Could you check a few things on this model? Use its own coordinates, in mm. A direction names the side the tool comes from. Coordinates: 2 decimals unless noted, no trailing zeros. Write each loop counter-clockwise with the first axis right and the second up, starting at its lowest first coordinate (ties: lowest second). Pieces come first, ordered by that corner, then holes.
Item 1: I want a section at A-A on x = 0. Please give me the cut outline in (y, z).
Item 2: I want a section at C-C on y = -30. Please give me the cut outline in (x, z), then the cut area to 3 significant figures.
Item 3: I want a section at D-D on x = 7.5. Please give me the cut outline in (y, z).
Item 4: For P1, Ø4, axis at x = -1.5, y = -21.5, coming from the -Z side; P2, Ø1.5, axis at y = -29.5, z = 0, coming from the -X side; P3, Ø10, axis at y = -20, z = 7.5, coming from the -X side, each with a flat end and sliding along its axis, tell me the tip position at first contact or that it passes through.
Item 5: Which directions (+Z, -Z, +X, -X, +Y, -Y) give clear straight access to the entire face, cutting with the end or side of a thin tool? Please do faces 1 (the flat face through (0, -35, 0)), 2 (the cylindrical face through (1.88, -24.86, -5.96)).
Item 6: If I drill on probe 1 along X at (y, z) = (-18, -0.25) (3 decimals); probe 2 along Y at (x, z) = (2, -4.25); probe 3 along Z at (x, y) = (-4.75, -1), over which ranges is the centre line in solid material (lowest first)?
Item 7: I want a section at B-B on z = 0. Please give me the cut outline in (x, y), then the cut area to 3 significant figures.
from build123d import *

# Parameters (mm, degrees)
SKETCH2_R           = 4
BOSS_EXTRUDE1_DEPTH = 15
SKETCH3_R           = 6.25
BOSS_EXTRUDE2_DEPTH = 20
FILLET1_R           = 10


with BuildPart() as part:
    # Sketch1 → Revolve1 (revolve)
    with BuildSketch(Plane.XY):
        with BuildLine():
            Line((0, 0), (0, 9.5))
            ThreePointArc((0, 9.5), (-9.5, 0), (0, -9.5))
            Line((0, -9.5), (0, 0))
        make_face()
    revolve(axis=Axis((0, 0, 0), (0, 1, 0)))

    # Sketch2 → Boss-Extrude1 (add)
    with BuildSketch(Plane(origin=(0, 0, 0), x_dir=(1, 0, 0), z_dir=(0, 1, 0))):
        with Locations(Location((0, 0, 0), (0, 0, 270))):
            Circle(SKETCH2_R)
    extrude(amount=-BOSS_EXTRUDE1_DEPTH)

    # Sketch3 → Boss-Extrude2 (add)
    with BuildSketch(Plane.XZ.offset(15)):
        with Locations(Location((0, 0, 0), (0, 0, 270))):
            Circle(SKETCH3_R)
    extrude(amount=BOSS_EXTRUDE2_DEPTH)

    # Fillet1
    # the kernel refuses this fillet: 10 mm, written as the material it adds along each edge
    with BuildSketch(Plane(origin=(0, -15, 0), x_dir=(0, 0, 1), z_dir=(-1, 0, 0))) as fillet1_piece_1:
        with BuildLine():
            CenterArc((14, 6.31961233), FILLET1_R, 180, 39.194967426)
            Line((4, 6.31961233), (3.8, 6.31961233))
            Line((3.8, 6.31961233), (3.8, 0))
            Line((3.8, 0), (4, -0.2))
            ThreePointArc((4, -0.2), (5.125, -0.2), (6.095, -0.126392247))
            Line((6.095, -0.126392247), (6.25, 0))
        make_face()
    revolve(axis=Axis((0, -15, 0), (0, 1, 0)))


solid = part.part
Response values:
1. outline: (-35, -6.25) - (-15, -6.25) arc R10 cw to (-8.68, -4) - (-8.62, -4) arc R9.5 ccw (long way) to (-8.62, 4) - (-8.68, 4) arc R10 cw to (-15, 6.25) - (-35, 6.25) - close
2. outline: circle Ø12.5 at (0, 0)
2. area: 123 mm2
3. outline: circle Ø11.66 at (0, 0)
4. P1: stops at z = -6.25
4. P2: stops at x = -6.25
4. P3: stops at x = -5.73
5. face 1: +Z, -Z, +X, -X, -Y
5. face 2: -Y
6. probe 1: x = -6.245 to 6.245
6. probe 2: y = -35 to -12.35, -8.26 to 8.26
6. probe 3: z = -8.17 to 8.17
7. outline: (-6.25, -35) - (6.25, -35) - (6.25, -15) arc R10 cw to (4, -8.68) - (4, -8.62) arc R9.5 ccw (long way) to (-4, -8.62) - (-4, -8.68) arc R10 cw to (-6.25, -15) - close
7. area: 589 mm2
